Geometry check sheet. Reference: the model listing, model coordinates, mm. Face numbers are marked on the shaded views. A direction names the side the tool comes from. Round coordinates to 2 decimals unless told otherwise and drop trailing zeros. Write each loop counter-clockwise with the first axis right and the second up, starting at its lowest first coordinate (ties: lowest second). Pieces come first, ordered by that corner, then holes.
Item 1: Cross-section at C-C (x = 90). Enter the section's corners in (y, z), then the cut area to 3 significant figures.
Item 2: Cross-section at B-B (y = 18). Enter the section's corners in (x, z), then the cut area to 3 significant figures.
Item 3: Depth check by flat-ended pin: P1, Ø5, axis at x = 157, z = -6, coming from the -Y side; P2, Ø12, axis at x = 63, z = 0.5, coming from the -Y side; P3, Ø1.5, axis at x = 156, z = 11, coming from the -Y side (3 decimals). Enter the tip coordinate at first touch or a pass-through.
Item 4: Cross-section at D-D (y = 48). Enter the section's corners in (x, z).
Item 5: Scan lines: probe 1 along Y at (x, z) = (215, 17.5); probe 2 along Y at (x, z) = (123.5, 12); probe 3 along Y at (x, z) = (98, -6.5). Record each from-to range of solid material in increasing order.
Item 6: Access from +Z, -Z, +X, -X, +Y, -Y to the whole of each face (thin tool, end or side, straight path). Record for the marked faces 4 and 5.
Item 7: Cross-section at A-A (z = -10.5). Enter the section's corners in (x, y), then the cut area to 3 significant figures.
Item 8: Draft check along X on the marked faces 1, 2 and 3. Enter one of: pulls with the +X half, pulls with the -X half, needs draft (parallel to the pull), parting line crosses it, or undercut.
from build123d import *

# Parameters (mm, degrees)
SALIENTE_EXTRUIR1_DEPTH = 20


with BuildPart() as part:
    # Croquis1 → Saliente-Extruir1 (new body, symmetric)
    with BuildSketch(Plane.XY):
        Polygon((130, 100), (0, 100), (12.328767123, 90), (113.117723961, 90), (124.520547945, 90), align=None)
        Polygon((12.328767123, 90), (0, 100), (0, 0), (90, 27), (80.603724142, 34.621423752), (69.015367917, 31.144916884), (10, 13.440306509), (10, 79.012937528), (10, 90), align=None)
        Polygon((80.603724142, 34.621423752), (12.328767123, 90), (10, 90), (10, 79.012937528), (69.015367917, 31.144916884), align=None)
        Polygon((124.520547945, 90), (113.117723961, 90), (83.200100156, 35.400336556), (96.846102629, 39.494137298), align=None)
        Polygon((83.200100156, 35.400336556), (80.603724142, 34.621423752), (90, 27), (96.846102629, 39.494137298), align=None)
        Polygon((96.846102629, 39.494137298), (90, 27), (250, 75), (229.461692114, 79.278814143), (209.367182815, 73.250461353), align=None)
        Polygon((250, 100), (130, 100), (178, 90), (240, 90), (240, 82.440306509), (229.461692114, 79.278814143), (250, 75), align=None)
        Polygon((178, 90), (130, 100), (124.520547945, 90), (128.969397311, 90), align=None)
    extrude(amount=SALIENTE_EXTRUIR1_DEPTH, both=True)


solid = part.part
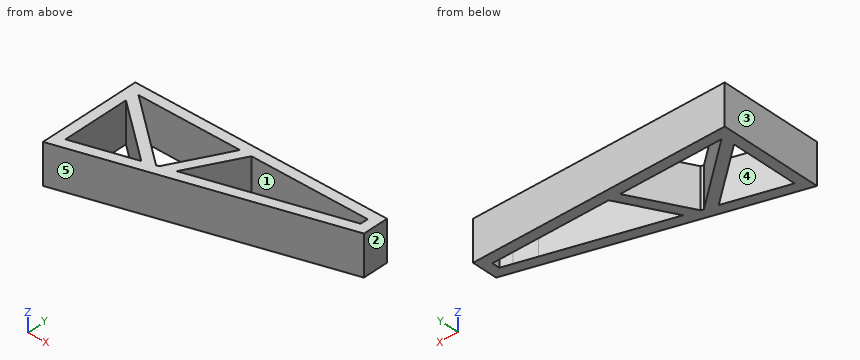
Resolved:
1. outline: (27, -20) - (47.81, -20) - (47.81, 20) - (27, 20) - close; (90, -20) - (100, -20) - (100, 20) - (90, 20) - close
1. area: 1,230 mm2
2. outline: (0, -20) - (10, -20) - (10, 20) - (0, 20) - close; (25.2, -20) - (60, -20) - (60, 20) - (25.2, 20) - close
2. area: 1,790 mm2
3. P1: stops at y = 46.35
3. P2: stops at y = 17.1
3. P3: stops at y = 46.575
4. outline: (0, -20) - (10, -20) - (10, 20) - (0, 20) - close; (48.24, -20) - (64.11, -20) - (64.11, 20) - (48.24, 20) - close; (90.1, -20) - (101.51, -20) - (101.51, 20) - (90.1, 20) - close; (125.2, -20) - (160, -20) - (160, 20) - (125.2, 20) - close
5. probe 1: y = 64.5 to 74.94, 90 to 100
5. probe 2: y = 37.05 to 47.49, 88.14 to 100
5. probe 3: y = 29.4 to 39.84, 41.6 to 62.41, 90 to 100
6. face 4: +Z, -Z
6. face 5: +Z, -Z, +X, -Y
7. outline: (0, 0) - (250, 75) - (250, 100) - (0, 100) - close; hole (10, 13.44) - (69.02, 31.14) - (10, 79.01) - close; hole (12.33, 90) - (80.6, 34.62) - (83.2, 35.4) - (113.12, 90) - close; hole (96.85, 39.49) - (240, 82.44) - (240, 90) - (124.52, 90) - close
7. area: 7,380 mm2
8. face 1: undercut
8. face 2: pulls with the +X half
8. face 3: pulls with the -X half
